Can you work these out from the model? Positions are in its coordinate system, mm. A direction names the side the tool comes from. Round coordinates to 2 decimals unless told otherwise and drop trailing zeros. Loops run counter-clockwise (first coordinate to the right, second up) from the corner with the lowest first, then second, coordinate; pieces in that order, holes last.
from build123d import *

# Parameters (mm, degrees)
BOSS_EXTRUDE1_DEPTH = 3.85


with BuildPart() as part:
    # Sketch1 → Boss-Extrude1 (new body)
    with BuildSketch(Plane.XY):
        Polygon((0, 5.646485633), (-4.89, 2.823242816), (-4.89, -2.823242816), (0, -5.646485633), (4.89, -2.823242816), (4.89, 2.823242816), align=None)
    extrude(amount=BOSS_EXTRUDE1_DEPTH)

    # Sketch2 → Revolve1 (revolve)
    with BuildSketch(Plane(origin=(0, 0, 0), x_dir=(0, 0, -1), z_dir=(1, 0, 0))):
        with BuildLine():
            Line((0, 0), (0, 3.25))
            ThreePointArc((0, 3.25), (0.073223305, 3.073223305), (0.25, 3))
            Line((0.25, 3), (149.5, 3))
            Line((149.5, 3), (150, 2.5))
            Line((150, 2.5), (150, 0))
            Line((150, 0), (0, 0))
        make_face()
    revolve(axis=Axis((0, 0, 0), (0, 0, -1)))

    # Sketch3 → Cut-Revolve1 (revolve, cut)
    with BuildSketch(Plane(origin=(0, 0, 0), x_dir=(0, 0, -1), z_dir=(1, 0, 0))):
        Polygon((-3.85, 5.646485633), (-3.413242816, 5.646485633), (-3.85, 4.89), align=None)
        Polygon((-0.15, 5.646485633), (-0.15, 4.53660254), (0, 4.45), (0, 5.646485633), align=None)
    revolve(axis=Axis((0, 0, 12.204941078), (0, 0, -1)), mode=Mode.SUBTRACT)


solid = part.part
(1) If we section it at A-A, the plane z = -67.5: List the corners of the cut face in (x, y) for me.
Worked answers:
outline: circle Ø6 at (0, 0)
(2) If I drill on line 1 (X direction, y = -1.75, z = -24); line 2 (Z direction, x = 1, y = -3.75); line 3 (Y direction, x = 1, z = -39), over which ranges is the centre line in solid material (lowest first)?
Worked answers:
line 1: x = -2.44 to 2.44
line 2: z = 0 to 3.85
line 3: y = -2.83 to 2.83
(3) For faces 1 (the flat face through (-2, -3, 0)), 2 (the conical face through (-4.385, -2.546, 3.746)), which set-ups out of +Z, -Z, +X, -X, +Y, -Y let a thin tool reach every point of the face, with its end or its side?
Worked answers:
face 1: -Z
face 2: +Z, -X, -Y
(4) Will these pins go through, and if not, where does the flat tip stop? P1, Ø2, axis at x = -0.5, z = -47, coming from the +Y side; P2, Ø3, axis at y = 0.5, z = -126.5, coming from the -X side; P3, Ø6, axis at y = -3.5, z = -21.5, coming from the +X side.
Worked answers:
P1: stops at y = 3
P2: stops at x = -3
P3: stops at x = 2.96
